```python
from build123d import *

# Parameters (mm, degrees)
SKETCH043_W             = 51
SKETCH043_H             = 2
SKETCH043_W_2           = 2
SKETCH043_H_2           = 51
PAD026_DEPTH            = 1.5
SKETCH044_R             = 4
SKETCH044_R_2           = 1.6
PAD027_DEPTH            = 2.7
HOLE001_D               = 3.4
HOLE001_DEPTH           = 25
HOLE001_CSINK_D         = 6.7
HOLE001_CSINK_ANGLE     = 90
BODY011_PLACEMENT_ANGLE = 180


with BuildPart() as part:
    # Sketch043 → Pad026 (new body)
    with BuildSketch(Plane.XY):
        with BuildLine():
            Line((-49.75, 40), (-49.75, -42))
            ThreePointArc((-49.75, -42), (-48.578427, -44.828427), (-45.75, -46))
            Line((-45.75, -46), (45.75, -46))
            ThreePointArc((45.75, -46), (48.578427, -44.828427), (49.75, -42))
            Line((49.75, -42), (49.75, 40))
            ThreePointArc((49.75, 40), (48.578427, 42.828427), (45.75, 44))
            Line((45.75, 44), (-45.75, 44))
            ThreePointArc((-45.75, 44), (-48.578427, 42.828427), (-49.75, 40))
        make_face()
        with Locations((0, 34)):
            Rectangle(SKETCH043_W, SKETCH043_H, mode=Mode.SUBTRACT)
        with Locations((0, -34)):
            Rectangle(SKETCH043_W, SKETCH043_H, mode=Mode.SUBTRACT)
        with Locations((36, 0)):
            Rectangle(SKETCH043_W_2, SKETCH043_H_2, mode=Mode.SUBTRACT)
        with Locations((-36, 0)):
            Rectangle(SKETCH043_W_2, SKETCH043_H_2, mode=Mode.SUBTRACT)
    extrude(amount=PAD026_DEPTH)

    # Sketch044 → Pad027 (join)
    with BuildSketch(Plane.XY):
        with Locations((-45.75, 40)):
            Circle(SKETCH044_R)
        with Locations((-45.75, 40)):
            Circle(SKETCH044_R_2, mode=Mode.SUBTRACT)
        with Locations((-30, 40)):
            Circle(SKETCH044_R)
        with Locations((-30, 40)):
            Circle(SKETCH044_R_2, mode=Mode.SUBTRACT)
        with Locations((30, 40)):
            Circle(SKETCH044_R)
        with Locations((30, 40)):
            Circle(SKETCH044_R_2, mode=Mode.SUBTRACT)
        with Locations((30, -42)):
            Circle(SKETCH044_R)
        with Locations((30, -42)):
            Circle(SKETCH044_R_2, mode=Mode.SUBTRACT)
        with Locations((-30, -42)):
            Circle(SKETCH044_R)
        with Locations((-30, -42)):
            Circle(SKETCH044_R_2, mode=Mode.SUBTRACT)
        with Locations((-45.75, -42)):
            Circle(SKETCH044_R)
        with Locations((-45.75, -42)):
            Circle(SKETCH044_R_2, mode=Mode.SUBTRACT)
        with Locations((45.75, -42)):
            Circle(SKETCH044_R)
        with Locations((45.75, -42)):
            Circle(SKETCH044_R_2, mode=Mode.SUBTRACT)
        with Locations((45.75, 40)):
            Circle(SKETCH044_R)
        with Locations((45.75, 40)):
            Circle(SKETCH044_R_2, mode=Mode.SUBTRACT)
    extrude(amount=PAD027_DEPTH)

    # Hole001
    with Locations(Plane(origin=(0, 0, 0), x_dir=(1, 0, 0), z_dir=(0, 0, -1))):
        with Locations((-45.75, -40), (-30, -40), (30, -40), (30, 42), (-30, 42), (-45.75, 42), (-45.75, 42), (-30, 42), (30, 42), (30, -40), (-30, -40), (-45.75, -40), (45.75, 42), (45.75, 42), (45.75, -40), (45.75, -40)):
            CounterSinkHole(HOLE001_D / 2, HOLE001_CSINK_D / 2, depth=HOLE001_DEPTH, counter_sink_angle=HOLE001_CSINK_ANGLE)


with BuildPart() as part_1:
    # Body011 placement: moved
    add(part.part.moved(Location((0, -1.8, 71.3))).rotate(Axis((0, -1.8, 71.3), (1, 0, 0)), BODY011_PLACEMENT_ANGLE))


solid = part_1.part
```
Check sheet for the modelled part. Datum: model origin and axes. Units: mm. A direction names the side the tool comes from. Round coordinates to 2 decimals unless told otherwise and drop trailing zeros. Loops run counter-clockwise (first coordinate to the right, second up) from the corner with the lowest first, then second, coordinate; pieces in that order, holes last. Notation, with made-up numbers: (72.5, 3) - (120.5, 3) arc R22 cw to (120.5, 38) - close; hole circle Ø11 at (-15, 46). An arc over 180 degrees is marked (long way). Answer as a JSON object with one key per item and string values. Group by question number.
Q1. Sectioned sample at C-C, the plane y = 27. Enter the section's corners in (x, z).
Q2. Mould release check, pull along Y, two halves, no side actions. Record for faces 3 (the face through (-1, -1, 69.8)), 4 (the face through (-28, 40, 68.6)): released by +Y, released by -Y, zero draft, split by the parting line, or undercut.
Q3. Set-up check for faces 1 (the face through (-30.521, 36.234, 69.208)), 2 (the face through (-30.8, -43.3, 69.1)): record each of +Z, -Z, +X, -X, +Y, -Y from which the full face is reachable in a straight line by a thin tool's end or side.
Q4. Gauge pin test, flat end, axial feed: P1, Ø5.5, axis at x = 45.75, y = 40.2, coming from the +Z side. Record the tip position at first contact, or that the pin passes through.
Q5. Sectioned sample at B-B, the plane x = 21. Enter the section's corners in (y, z), plus the area to 3 significant figures.
Q6. Scan lines: line 1 along Y through (x, z) = (-6.5, 70.05); line 2 along Y through (x, z) = (-45.75, 69.1); line 3 along X through (y, z) = (15.5, 70.7). Record each from-to range of solid material in increasing order. Write a range as [from, to].
Q7. Sectioned sample at A-A, the plane z = 70.3. Count the separate pieces of the cut face and the enclosed holes in it, plus the area to 3 significant figures.
Solution:
{
 "1": {"outline": "(-49.75, 69.8) - (49.75, 69.8) - (49.75, 71.3) - (-49.75, 71.3) - close"},
 "2": {"face 3": "undercut", "face 4": "zero draft"},
 "3": {"face 1": "-Z", "face 2": "+Z, -Z"},
 "4": {"P1": "stops at z = 70.7"},
 "5": {"outline": "(-45.8, 69.8) - (-36.8, 69.8) - (-36.8, 71.3) - (-45.8, 71.3) - close; (-34.8, 69.8) - (31.2, 69.8) - (31.2, 71.3) - (-34.8, 71.3) - close; (33.2, 69.8) - (44.2, 69.8) - (44.2, 71.3) - (33.2, 71.3) - close", "area": "129 mm²"},
 "6": {"line 1": "y = [-45.8, -36.8], [-34.8, 31.2], [33.2, 44.2]", "line 2": "y = [-45.8, -43.5], [-40.1, -37.8], [36.2, 38.5], [41.9, 44.2]", "line 3": "x = [-49.75, -37], [-35, 35], [37, 49.75]"},
 "7": {"separate pieces": "1", "enclosed holes": "12", "area": "8,390 mm²"}
}
